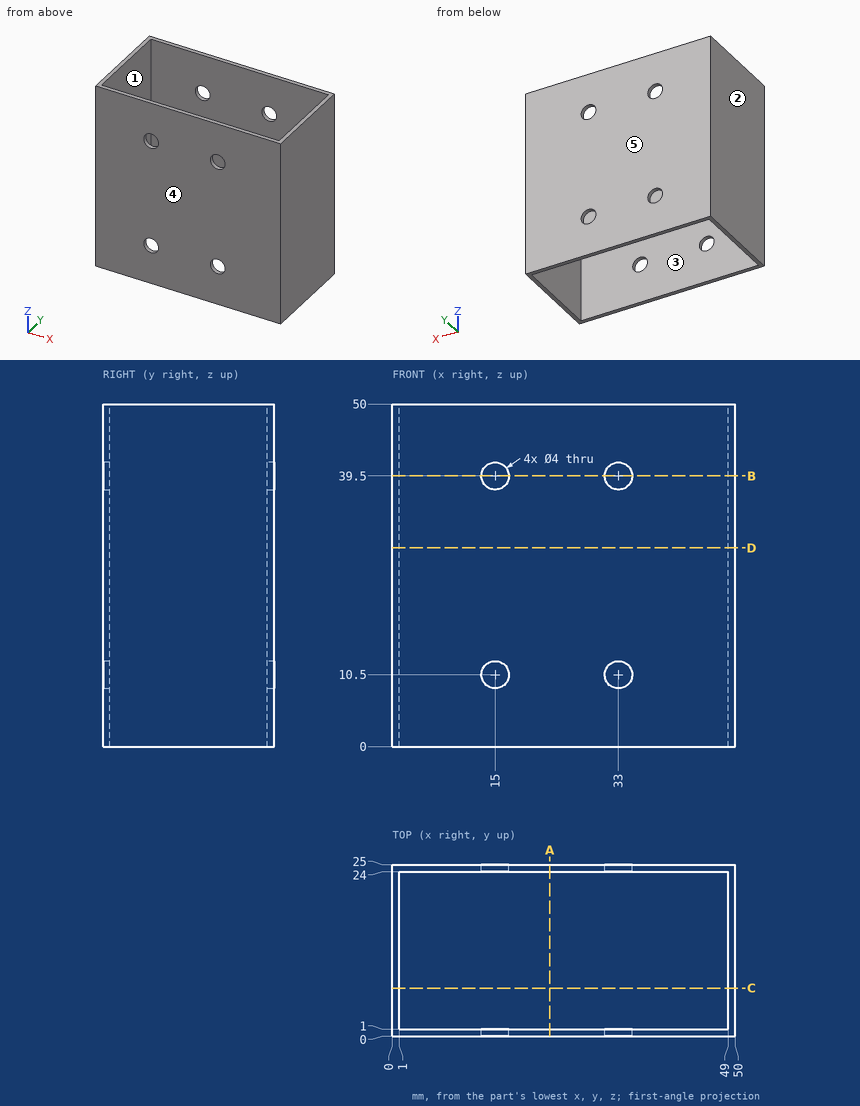
Geometry: see drawing. Coordinates: mm, zero at the bounding-box minimum. A direction names the side the tool comes from. Give positions to 0.01 mm unless a question says otherwise; leave off trailing zeros. Write each loop counter-clockwise with the first axis right and the second up, starting at its lowest first coordinate (ties: lowest second). Pieces come first, ordered by that corner, then holes. Notation, with made-up numbers: M 28,28.5 L 75,28.5 A28 cw 75,65.5 Z; hole C 30.25,-21 d4. An arc over 180 degrees is marked long. Answer in a Markdown table with one row per item. Add a question column.
(1) Section A-A on x = 23. Return loops of the section in (y, z), and give its area (3 significant figures).
(2) First-contact query: pin 1 (4.5 mm diameter, centred on x = 15, z = 39.5, fed in from +Y). Flat tip, straight axial feed; report the tip coordinate or a pass-through.
(3) Reachability of the marked faces 1 and 2 from +Z, -Z, +X, -X, +Y, -Y: full face, straight path, thin tool, end or side. Return the list, or none.
(4) Ray query, line 1 (X direction, y = 24.7, z = 39.5); line 2 (Y direction, x = 39.5, z = 25); line 3 (X direction, y = 13, z = 34). Return the intervals inside material, ascending.
(5) Mould query, pull axis Y, two halves, no side actions, for the marked faces 3, 4 and 5. Classes: +Y half, -Y half, draft (parallel to the pull), parting line (faces both ways), or undercut.
(6) Section B-B on z = 39.5. Return loops of the section in (x, y), and give its area (3 significant figures).
(7) Section C-C on y = 7. Return loops of the section in (x, z), and give its area (3 significant figures).
(8) Section D-D on z = 29. Return loops of the section in (x, y).
Result set:
| question | item | result |
|---|---|---|
| 1 | outline | M 0,0 L 1,0 L 1,50 L 0,50 Z; M 24,0 L 25,0 L 25,50 L 24,50 Z |
| 1 | area | 100 mm^2 |
| 2 | pin 1 | stops at y = 25 |
| 3 | face 1 | +Z, -Z |
| 3 | face 2 | +Z, -Z, -X, +Y, -Y |
| 4 | line 1 | x = 0 to 13, 17 to 31, 35 to 50 |
| 4 | line 2 | y = 0 to 1, 24 to 25 |
| 4 | line 3 | x = 0 to 1, 49 to 50 |
| 5 | face 3 | undercut |
| 5 | face 4 | -Y half |
| 5 | face 5 | +Y half |
| 6 | outline | M 0,0 L 13,0 L 13,1 L 1,1 L 1,24 L 13,24 L 13,25 L 0,25 Z; M 17,0 L 31,0 L 31,1 L 17,1 Z; M 17,24 L 31,24 L 31,25 L 17,25 Z; M 35,0 L 50,0 L 50,25 L 35,25 L 35,24 L 49,24 L 49,1 L 35,1 Z |
| 6 | area | 130 mm^2 |
| 7 | outline | M 0,0 L 1,0 L 1,50 L 0,50 Z; M 49,0 L 50,0 L 50,50 L 49,50 Z |
| 7 | area | 100 mm^2 |
| 8 | outline | M 0,0 L 50,0 L 50,25 L 0,25 Z; hole M 1,1 L 49,1 L 49,24 L 1,24 Z |
